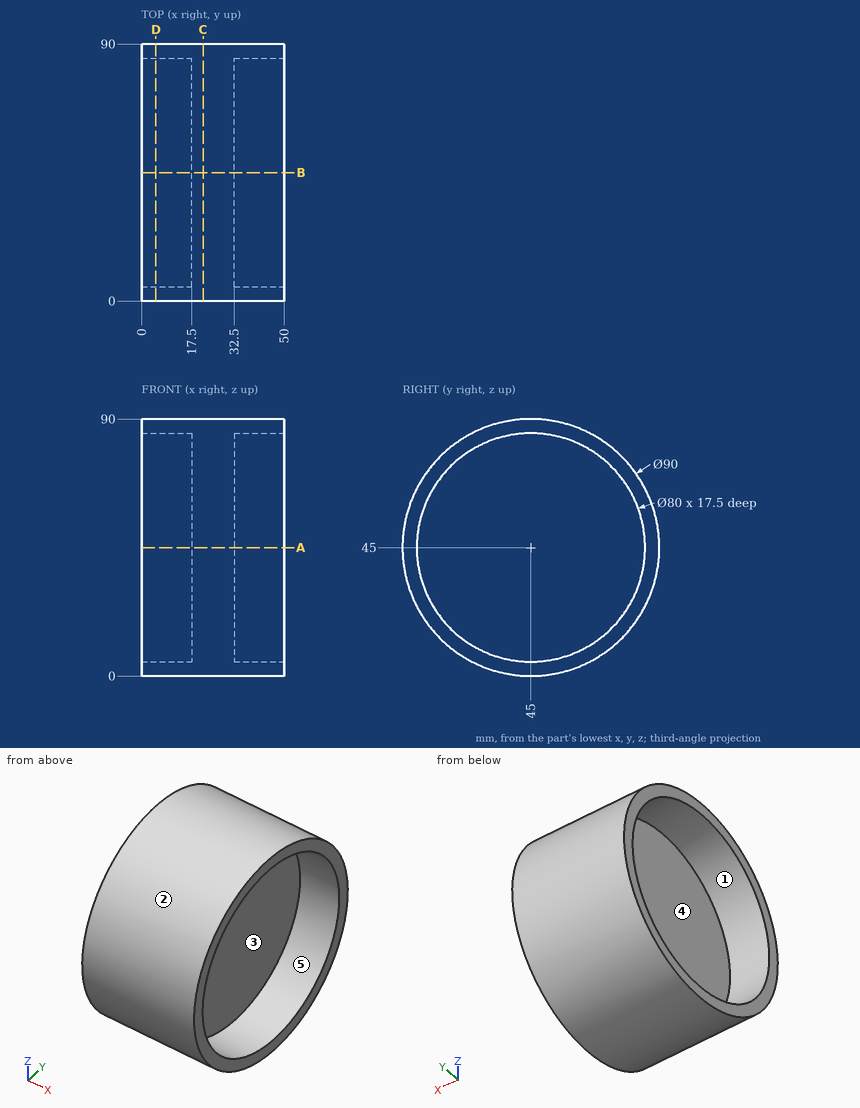
Input: dimensioned drawing with shaded views. Units: mm. Origin: part minimum x, y, z. A direction names the side the tool comes from. Coordinates: 2 decimals unless noted, no trailing zeros. Loops run counter-clockwise (first coordinate to the right, second up) from the corner with the lowest first, then second, coordinate; pieces in that order, holes last. Notation, with made-up numbers: M 20,-40 L 74,-40 A30 cw 74,-8 Z; hole C 15.25,3.5 d7. An arc over 180 degrees is marked long. One line per item, written item: value. Start each with the question number.
1) Cut plane A-A (z = 45). Return loops of the section in (x, y).
2) Draft query along Z for the marked faces 1, 2 and 3. Return one class per face: released by +Z, released by -Z, zero draft, split by the parting line, or undercut.
3) Material intervals for L1, parallel to Z at x = 9, y = 45; L2, parallel to X at y = 35, z = 66.5, sorted ascending. Write a range as from..to.
4) Pin query (flat end, axial travel): P1, Ø5, axis at y = 27.5, z = 80.5, coming from the +X side; P2, Ø2, axis at y = 74.5, z = 33.5, coming from the +X side; P3, Ø5, axis at y = 71.5, z = 23.5, coming from the -X side; P4, Ø12, axis at x = 26.5, z = 80, coming from the +Y side. Return the tip coordinate at first contact, or that it passes through.
5) Reachability of the marked faces 4 and 5 from +Z, -Z, +X, -X, +Y, -Y: full face, straight path, thin tool, end or side. Return the list, or none.
6) Cut plane C-C (x = 21.5). Return loops of the section in (y, z).
7) Cut plane D-D (x = 5). Return loops of the section in (y, z).
Evaluation:
1. outline: M 0,0 L 50,0 L 50,5 L 32.5,5 L 32.5,85 L 50,85 L 50,90 L 0,90 L 0,85 L 17.5,85 L 17.5,5 L 0,5 Z
2. face 1: undercut
2. face 2: split by the parting line
2. face 3: undercut
3. L1: 0..5, 85..90
3. L2: 17.5..32.5
4. P1: x = 50
4. P2: x = 32.5
4. P3: x = 17.5
4. P4: y = 79.41
5. face 4: -X
5. face 5: +X
6. outline: C 45,45 d90
7. outline: C 45,45 d90; hole C 45,45 d80
